from build123d import *

# Parameters (mm, degrees)
SKETCH1_W           = 130
SKETCH1_H           = 130
BOSS_EXTRUDE1_DEPTH = 50
SKETCH2_W           = 120
SKETCH2_H           = 120
CUT_EXTRUDE1_DEPTH  = 45
SKETCH3_R           = 2.5
BOSS_EXTRUDE2_DEPTH = 5


with BuildPart() as part:
    # Sketch1 → Boss-Extrude1 (new body)
    with BuildSketch(Plane(origin=(0, 0, 0), x_dir=(1, 0, 0), z_dir=(0, 1, 0))):
        with Locations((65, 65)):
            Rectangle(SKETCH1_W, SKETCH1_H)
    extrude(amount=BOSS_EXTRUDE1_DEPTH)

    # Sketch2 → Cut-Extrude1 (cut)
    with BuildSketch(Plane.XZ):
        with Locations((65, -65)):
            Rectangle(SKETCH2_W, SKETCH2_H)
    extrude(amount=-CUT_EXTRUDE1_DEPTH, mode=Mode.SUBTRACT)

    # Sketch3 → Boss-Extrude2 (add)
    with BuildSketch(Plane(origin=(0, 45, 0), x_dir=(-1, 0, 0), z_dir=(0, -1, 0))):
        with Locations((-9, 121)):
            Circle(SKETCH3_R)
        with Locations((-121, 121)):
            Circle(SKETCH3_R)
        with Locations((-9, 9)):
            Circle(SKETCH3_R)
        with Locations((-121, 9)):
            Circle(SKETCH3_R)
    extrude(amount=BOSS_EXTRUDE2_DEPTH)


solid = part.part
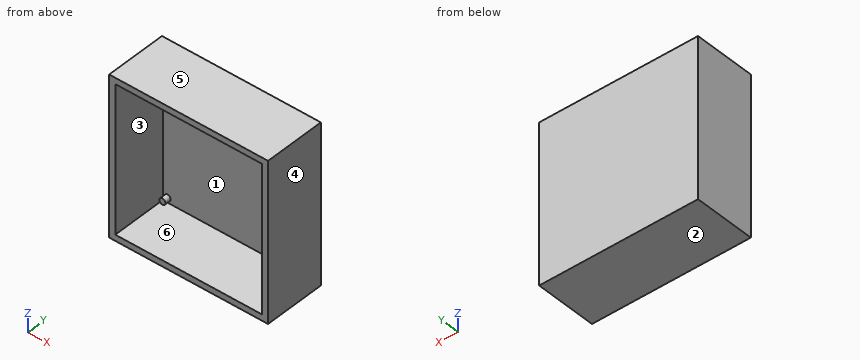
Can you work these out from the model? Positions are in its coordinate system, mm. Face numbers are marked on the shaded views. A direction names the side the tool comes from. Give positions to 0.01 mm unless a question says otherwise; leave off trailing zeros. Write each loop counter-clockwise with the first axis right and the second up, starting at its lowest first coordinate (ties: lowest second). Pieces come first, ordered by that corner, then holes. Notation, with made-up numbers: (-27.5, -37.5) -> (5.5, -37.5) arc R20 cw to (5.5, -6.5) -> close; hole circle Ø2 at (23, -37). An arc over 180 degrees is marked (long way). Answer as a JSON object with one key per item and string values. Group by question number.
Item 1: Suppose I cut it at B-B (z = -90). Please give me the cut outline in (x, y).
Item 2: Please list where these lines run through material, in increasing order: line 1 (X direction, y = 8, z = -93); line 2 (Z direction, x = 97, y = 6); line 3 (Y direction, x = 118, z = -122). Write a range as [from, to].
Item 3: I'm going to push flat-ended pins straight in: P1, Ø6, axis at x = 20.5, z = -91.5, coming from the -Y side; P2, Ø5.5, axis at x = 122, z = -120.5, coming from the -Y side. Where does each tip first touch, or does it pass through?
Item 4: We'd pull the mould along Z, two halves only. Please class the marked faces 3, 4, 5 and 6: +Z half, -Z half, draft (parallel to the pull), parting line (faces both ways), or undercut.
Item 5: Suppose I cut it at D-D (x = 121). Please give me the cut outline in (y, z).
Item 6: Suppose I cut it at C-C (x = 16). Please give me the cut outline in (y, z).
Item 7: Suppose I cut it at A-A (y = 16.5). Please give me the cut outline in (x, z), plus the area to 3 significant figures.
Item 8: For the marked faces 1 and 2, which set-ups out of +Z, -Z, +X, -X, +Y, -Y let a thin tool reach every point of the face, with its end or its side?
Findings:
{
 "1": {"outline": "(0, 0) -> (5, 0) -> (5, 45) -> (125, 45) -> (125, 0) -> (130, 0) -> (130, 50) -> (0, 50) -> close"},
 "2": {"line 1": "x = [0, 5], [125, 130]", "line 2": "z = [-130, -125], [-5, 0]", "line 3": "y = [45, 50]"},
 "3": {"P1": "stops at y = 45", "P2": "stops at y = 40"},
 "4": {"face 3": "undercut", "face 4": "draft", "face 5": "+Z half", "face 6": "undercut"},
 "5": {"outline": "(0, -130) -> (50, -130) -> (50, 0) -> (0, 0) -> (0, -5) -> (45, -5) -> (45, -6.5) -> (40, -6.5) -> (40, -11.5) -> (45, -11.5) -> (45, -118.5) -> (40, -118.5) -> (40, -123.5) -> (45, -123.5) -> (45, -125) -> (0, -125) -> close"},
 "6": {"outline": "(0, -130) -> (50, -130) -> (50, 0) -> (0, 0) -> (0, -5) -> (45, -5) -> (45, -125) -> (0, -125) -> close"},
 "7": {"outline": "(0, -130) -> (130, -130) -> (130, 0) -> (0, 0) -> close; hole (5, -125) -> (125, -125) -> (125, -5) -> (5, -5) -> close", "area": "2,500 mm²"},
 "8": {"face 1": "-Y", "face 2": "-Z, +X, -X, +Y, -Y"}
}
